Geometry check sheet. Reference: the model listing, model coordinates, mm. A direction names the side the tool comes from. Coordinates: 2 decimals unless noted, no trailing zeros. Order: outer loops, then holes, each group sorted by start corner. A loop starts at its lowest first (then second) coordinate and runs counter-clockwise, first axis right, second up. Notation, with made-up numbers: M -22,13.5 L 2,13.5 A18 cw 2,41.5 Z; hole C 64,30.25 d7. An arc over 180 degrees is marked long. One line per item, written item: value. Start each with the question number.
1) Sectioned sample at C-C, the plane z = -13. Enter the section's corners in (x, y).
2) Sectioned sample at D-D, the plane z = -7. Enter the section's corners in (x, y), then the cut area to 3 significant figures.
3) Access from +Z, -Z, +X, -X, +Y, -Y to the whole of each face (thin tool, end or side, straight path). Record for faces 1 (the flat face through (-4, 15.5, -11.665)), 2 (the flat face through (12.3, 14.1, -18.465)).
4) Sectioned sample at A-A, the plane y = 0. Enter the section's corners in (x, z).
5) Draft check along X on faces 3 (the cylindrical face through (-13.887, 10.648, -14.525)), 4 (the cylindrical face through (-23.977, -1.055, -12.155)), 5 (the flat face through (-5, 16, -5.665)). Enter one of: pulls with the +X half, pulls with the -X half, needs draft (parallel to the pull), parting line crosses it, or undercut.
6) Go/stop test with flat-tipped pins: P1, Ø3, axis at y = 10.5, z = -16, coming from the -X side; P2, Ø3, axis at x = 18.5, z = -11, coming from the +Y side; P3, Ø4, axis at x = -7.5, y = 13.5, coming from the -Z side. Record where each tip stops, or that it passes through.
7) Thickness scan on L1, parallel to Y at x = 0, z = -13.9; L2, parallel to X at y = 0, z = -8. Record the ranges inside material, lowest first. Write a range as from..to.
```python
from build123d import *

# Parameters (mm, degrees)
CHANFREIN2_SIZE = 1


with BuildPart() as part:
    # Esquisse1 → Révolution1 (revolve)
    with BuildSketch(Plane(origin=(0, 0, 0), x_dir=(1, 0, 0), z_dir=(0, 1, 0))):
        Polygon((24, 5.665131579), (24, 18.465131579), (17.5, 18.465131579), (17.5, 11.665131579), (15.7, 11.665131579), (15.7, 5.665131579), align=None)
    revolve(axis=Axis((0, 0, 0), (0, 0, -1)))

    # Chanfrein2
    chanfrein2_edges = [part.edges().sort_by_distance(p)[0] for p in [
        (-17.5, 0, -18.465131579),
    ]]
    chamfer(chanfrein2_edges, length=CHANFREIN2_SIZE)


solid = part.part
```
Final values:
1. outline: C 0,0 d48; hole C 0,0 d35
2. outline: C 0,0 d48; hole C 0,0 d31.4
2. area: 1,040 mm^2
3. face 1: -Z
3. face 2: -Z, +X, -X, +Y, -Y
4. outline: M -24,-18.47 L -18.5,-18.47 L -17.5,-17.47 L -17.5,-11.67 L -15.7,-11.67 L -15.7,-5.67 L -24,-5.67 Z; M 15.7,-11.67 L 17.5,-11.67 L 17.5,-17.47 L 18.5,-18.47 L 24,-18.47 L 24,-5.67 L 15.7,-5.67 Z
5. face 3: undercut
5. face 4: parting line crosses it
5. face 5: needs draft
6. P1: stops at x = -22.25
6. P2: stops at y = 16.94
6. P3: stops at z = -11.67
7. L1: y = -24..-17.5, 17.5..24
7. L2: x = -24..-15.7, 15.7..24
